```python
from build123d import *

# Parameters (mm, degrees)
F1_DEPTH = 32
F2_R     = 5.5
F3_DEPTH = 13.001
F5_DEPTH = 19
F4_R     = 6.5
F6_DEPTH = 88.001
F8_DEPTH = 19


with BuildPart() as f1:
    # F0 (on Front) → F1 (new body)
    with BuildSketch(Plane.XZ):
        Polygon((25, 0), (0, 0), (0, -13), (39, -13), (39, 4), (74, 4), (74, -13), (113, -13), (113, 0), (88, 0), (88, 43.748), (69, 43.748), (69, 17), (44, 17), (44, 43.748), (25, 43.748), align=None)
    extrude(amount=F1_DEPTH)

    # F2 (on Top) → F3 (cut, through all)
    with BuildSketch(Plane.XY):
        with Locations((13, -13)):
            Circle(F2_R)
        with Locations((100.350889, -13)):
            Circle(F2_R)
        Polygon((16, -32), (0, -16), (0, -32), align=None)
        Polygon((113, -22), (103, -32), (113, -32), align=None)
    extrude(amount=-F3_DEPTH, mode=Mode.SUBTRACT)

    # F4 (on face) → F5 (join)
    with BuildSketch(Plane(origin=(25, 0, 0), x_dir=(0, -1, 0), z_dir=(-1, 0, 0))):
        with BuildLine():
            ThreePointArc((32, 43.748), (16, 48.035187), (0, 43.748))
            Line((0, 43.748), (32, 43.748))
        make_face()
    extrude(amount=-F5_DEPTH)

    # F4 (on face) → F6 (cut, through all)
    with BuildSketch(Plane(origin=(25, 0, 0), x_dir=(0, -1, 0), z_dir=(-1, 0, 0))):
        with Locations((16, 33)):
            Circle(F4_R)
    extrude(amount=-F6_DEPTH, mode=Mode.SUBTRACT)

    # F7 (on face) → F8 (join)
    with BuildSketch(Plane.YZ.offset(88)):
        with BuildLine():
            ThreePointArc((0, 43.748), (-16, 48.035187), (-32, 43.748))
            Line((-32, 43.748), (0, 43.748))
        make_face()
    extrude(amount=-F8_DEPTH)


solid = f1.part
```
Input: part model. Units: mm. Frame: model coordinates. A direction names the side the tool comes from. Coordinates: 2 decimals unless noted, no trailing zeros. Write each loop counter-clockwise with the first axis right and the second up, starting at its lowest first coordinate (ties: lowest second). Pieces come first, ordered by that corner, then holes.
1) Section C-C on z = 41.5. Output: boundary loops of the cut face in (x, y).
2) Section A-A on z = -3. Output: boundary loops of the cut face in (x, y), and give its area (3 significant figures).
3) Mould query, pull axis X, two halves, no side actions, for faces 1 (the flat face through (0, -8, -6)), 2 (the flat face through (57, -16, 17)), 3 (the flat face through (101, -19, 0)). Classes: pulls with the +X half, pulls with the -X half, needs draft (parallel to the pull), parting line crosses it, or undercut.
4) Section D-D on y = -13. State how many separate pieces and enclosed holes the cut face has, and give its area (3 significant figures).
5) Pin query (flat end, axial travel): pin 1 Ø1.5 at (y, z) = (-17.5, 40) entering from +X; pin 2 Ø12 at (y, z) = (-18.5, 9.5) entering from -X; pin 3 Ø8 at (x, y) = (86.5, -21) entering from +Z; pin 4 Ø9 at (x, y) = (13, -13) entering from +Z. Return the tip coordinate at first contact, or that it passes through.
6) Set-up query: faces 4 (the flat face through (56, -16, 4)), 5 (the flat face through (69, -16, 26)), 6 (the cylindrical face through (78.633, -15.765, 48.034)), 7 (the flat face through (88, -16, 24)), 8 (the cylindrical face through (78.367, -11.209, 37.393)). Return all of +Z, -Z, +X, -X, +Y, -Y with unobstructed straight access to the full face (end or side cutting, diameter ignored); none if empty.
7) Section B-B on x = 13. Output: boundary loops of the cut face in (y, z), and give its area (3 significant figures).
8) Material intervals for line 1 along X through (y, z) = (-1.5, -9); line 2 along X through (y, z) = (-3, 43); line 3 along X through (y, z) = (-14, -8), sorted ascending.
Check result:
1. outline: (25, -32) - (44, -32) - (44, 0) - (25, 0) - close; (69, -32) - (88, -32) - (88, 0) - (69, 0) - close
2. outline: (0, -16) - (16, -32) - (39, -32) - (39, 0) - (0, 0) - close; (74, -32) - (103, -32) - (113, -22) - (113, 0) - (74, 0) - close; hole circle Ø11 at (13, -13); hole circle Ø11 at (100.35, -13)
2. area: 2,130 mm2
3. face 1: pulls with the -X half
3. face 2: undercut
3. face 3: needs draft
4. separate pieces: 5
4. enclosed holes: 0
4. area: 2,390 mm2
5. pin 1: stops at x = 88
5. pin 2: stops at x = 25
5. pin 3: stops at z = 48.02
5. pin 4: passes through
6. face 4: -Z, +Y, -Y
6. face 5: +Z, +Y, -Y
6. face 6: +Z, +X, -X
6. face 7: +Z, +X, +Y, -Y
6. face 8: +X, -X
7. outline: (-29, -13) - (-18.5, -13) - (-18.5, 0) - (-29, 0) - close; (-7.5, -13) - (0, -13) - (0, 0) - (-7.5, 0) - close
7. area: 234 mm2
8. line 1: x = 0 to 39, 74 to 113
8. line 2: x = 25 to 44, 69 to 88
8. line 3: x = 0 to 7.59, 18.41 to 39, 74 to 94.94, 105.76 to 113
